Autodesk Inventor part; units mm, degrees
ref_plane "Work Plane1" through (29, 0, 0) normal (0, -1, 0) x (1, 0, 0)
ref_plane "YZ Plane" through (0, 0, 0) normal (1, 0, 0) x (0, 1, 0)
ref_plane "XZ Plane" through (0, 0, 0) normal (0, 1, 0) x (-1, 0, 0)
sketch "Sketch1" plane through (0, 0, 0) normal (0, 0, 1) x (1, 0, 0)
  line L0 (0.2709, 0) -> (6.35, 0)
  line L1 (6.35, 0) -> (6.35, 2.413)
  line L2 (6.35, 2.413) -> (2.1084, 2.413)
  line L3 (2.1084, 2.413) -> (0.0001, 2.413)
  line L4 (0.0001, 2.413) -> (0, 2.413)
  line L5 (0, 2.413) -> (0, 4.5847)
  line L6 (0, 4.5847) -> (-2.5654, 4.5847)
  line L7 (-2.5654, 4.5847) -> (-2.5654, 1.8331)
  line L8 (-2.5654, 1.8331) -> (-0.7874, 1.8331)
  line L9 (-0.7874, 1.8331) -> (0.2709, 0)
  line L10 (-4.3485, 0) -> (8.1331, 0)
  line L11 (0, -0.9169) -> (0, 5.5016)
  line L12 (2.1084, 2.413) -> (0, 2.413) construction
  dimension "d1" = 4.2416
  dimension "d2" = 2.1083
  dimension "d3" = 2.5654
  dimension "d4" = 1.778
  dimension "d5" = 60
  dimension "d6" = 4.826
  dimension "d7" = 4.826
  dimension "d8" = 3.6662
  dimension "d9" = 9.1694
  dimension "d26" = 6.35
revolve "Body" add sketch "Sketch1" angle 360 about axis through (0.2709, 0, 0) along (1, 0, 0) contours L9 L11 L3 L2 L1 L0 | L9 L8 L7 L6 L5 L11
sketch "Sketch2" plane through (-2.5654, 0, 0) normal (-1, 0, 0) x (0, 0, 1)
  circle A0 centre (0, 0) radius 1.8331
  line L0 (0, -6.4186) -> (0, 6.4186)
  line L1 (-6.4186, 0) -> (6.4186, 0)
  line L2 (1.8331, 0) -> (0.9165, -1.5875)
  line L3 (0.9165, -1.5875) -> (-0.9165, -1.5875)
  line L4 (-0.9165, -1.5875) -> (-1.8331, 0)
  line L5 (-1.8331, 0) -> (-0.9165, 1.5875)
  line L6 (-0.9165, 1.5875) -> (0.9165, 1.5875)
  line L7 (0.9165, 1.5875) -> (1.8331, 0)
  point P0 (0, 0)
extrude "Slot" add sketch "Sketch2" against normal up to next contours L7 A0 | A0 L2 | L6 L0 A0 | A0 L0 L3 | L0 L6 A0 | A0 L3 L0 | L4 A0 | A0 L5
fillet "Fillet1" radius 2.3114 1 edges at (-2.5654, -4.5847, 0)
thread "Thread"
chamfer "Chamfer1" distance 0.6492 distance2 0.6492 1 edges at (6.35, -2.413, 0) measured on face at (6.35, -0.2686, 0.7084)
ref_plane "Work Plane1" through (29, 0, 0) normal (0, -1, 0) x (1, 0, 0)
fillet "Fillet2" radius 0.1 1 edges at (0.0001, -2.413, 0)
equation "\"d30\" = R"
equation "\"d17\" = RR"
equation "\"d13\" = GEL"
equation "\"d15\" = -0.5 * SPD + 0.5 * GD"
equation "\"d16\" = GUL"
equation "\"d1\" = GEL"
equation "\"d3\" = KOH"
equation "\"d4\" = INTI"
equation "\"d6\" = GD"
equation "\"d7\" = BDM"
equation "\"d8\" = 1.1547 * SW"
equation "\"d9\" = KOD"
equation "\"d26\" = NLG"
equation "\"GD\" = NND"
equation "\"NLG\" = 6.35"
equation "\"GEL\" = 4.2416"
equation "\"KOD\" = 9.1694"
equation "\"KOH\" = 2.5654"
equation "\"INTI\" = 1.778"
equation "\"GAL\" = 2.1082"
equation "\"GUL\" = 0.64922"
equation "\"BDM\" = NND"
equation "\"SW\" = 3.175"
equation "\"RR\" = 2.3114"
equation "\"SPD\" = 3.52755"
equation "\"R\" = 0.1"
equation "\"TOA\" = 30deg"
equation "\"GD1\" = SPD"
equation "\"THREADDIA\" = 4.826"
equation "\"KOH1\" = 0.508"
equation "\"NND\" = 4.826"
equation "\"E0\" = 3.66725"
properties part number "ANSI B18.3 - 10 - 24 x 1/4, HSBHCSI" material "Steel, Mild"
The model under review builds one solid part; all positions refer to its coordinate system, in mm. A direction names the side the tool comes from. Give positions to 0.01 mm unless a question says otherwise; leave off trailing zeros. Loops run counter-clockwise (first coordinate to the right, second up) from the corner with the lowest first, then second, coordinate; pieces in that order, holes last. Notation, with made-up numbers: (-30.75, 88) - (27.25, 88) arc R23 ccw to (27.25, 96) - close; hole circle Ø11 at (-19.5, 29). An arc over 180 degrees is marked (long way). Answer as a JSON object with one key per item and string values.
Q1. Add section A-A on x = 1. State the section outline as (y, z) points.
Worked out:
{"outline": "circle Ø4.83 at (0, 0)"}
Q2. Mouldability with a two-part tool opening along Y and no side actions: class faces 1 (the cylindrical face through (2.861, -1.915, 1.468)), 2 (the flat face through (-2, -1.588, 0)), 3 (the flat face through (6.35, 0, 0)) as +Y half, -Y half, draft (parallel to the pull), parting line (faces both ways), or undercut.
Worked out:
{"face 1": "parting line", "face 2": "undercut", "face 3": "draft"}
Q3. To check wall thickness, follow line 1 along Z through (x, y) = (-0.75, -0.25); line 2 along Z through (x, y) = (-0.75, -1); line 3 along Y through (x, z) = (6, -1). State the ranges of each line that lie inside material, in increasing order.
Worked out:
{"line 1": "z = -4.52 to -1.69, 1.69 to 4.52", "line 2": "z = -4.42 to -1.26, 1.26 to 4.42", "line 3": "y = -1.86 to 1.86"}
Q4. Insertion check: pin 1 (2 mm diameter, centred on x = -2, z = 0, fed in from +Y); pin 2 (4 mm diameter, centred on x = -0.5, y = -2.5, fed in from -Z); pin 3 (4 mm diameter, centred on x = 4, y = -0.5, fed in from +Z). Each pin has a flat end and moves straight along its axis. Give the tip position at first contact, or say it passes through.
Worked out:
{"pin 1": "stops at y = 4.46", "pin 2": "stops at z = -4.56", "pin 3": "stops at z = 2.41"}
Q5. For faces 4 (the flat face through (-2.565, -2, 0)), 5 (the conical face through (0, -1, 3)), 6 (the flat face through (-2, 1.588, 0)), list the 3-axis set-ups (+Z, -Z, +X, -X, +Y, -Y) from which the entire face can be reached by the end or side of a thin tool; tool diameter is ignored.
Worked out:
{"face 4": "+Z, -Z, -X, +Y, -Y", "face 5": "+X", "face 6": "-X"}
